```python
from build123d import *

# Parameters (mm, degrees)
F0_W     = 30
F0_H     = 30
F0_R     = 5
F1_DEPTH = 3
F0_R_2   = 4
F2_DEPTH = 6.5
F3_DEPTH = 13.5
F5_D     = 5


with BuildPart() as f1:
    # F0 (on Top) → F1 (new body)
    with BuildSketch(Plane.XY):
        Rectangle(F0_W, F0_H)
        Circle(F0_R, mode=Mode.SUBTRACT)
    extrude(amount=F1_DEPTH)

    # F0 (on Top) → F2 (join)
    with BuildSketch(Plane.XY):
        Circle(F0_R)
        Circle(F0_R_2, mode=Mode.SUBTRACT)
    extrude(amount=F2_DEPTH)

    # F0 (on Top) → F3 (join)
    with BuildSketch(Plane.XY):
        Circle(F0_R_2)
    extrude(amount=F3_DEPTH)

    # F5 (through all)
    with Locations(Plane.XY.offset(3)):
        with Locations((8.5, 8.5), (-8.5, 8.5), (-8.5, -8.5), (8.5, -8.5)):
            Hole(F5_D / 2)


with BuildPart() as f6_1:
    # F6: copy of F1
    add(f1.part.moved(Location((50, 0, 0))))


solid = f1.part
```
Read the model definition and answer for the solid it produces. Units are mm, in the model's axes. A direction names the side the tool comes from. Coordinates: 2 decimals unless noted, no trailing zeros. Loops run counter-clockwise (first coordinate to the right, second up) from the corner with the lowest first, then second, coordinate; pieces in that order, holes last. Notation, with made-up numbers: (52.5, -4.5) -> (59.5, -4.5) arc R22 cw to (59.5, 21.5) -> close; hole circle Ø10 at (-16, 30). An arc over 180 degrees is marked (long way). Return JSON: item names as keys, results as strings.
Item 1: Find section C-C (z = 1.25). Determine the outline of the cut face in (x, y).
Answers:
{"outline": "(-15, -15) -> (15, -15) -> (15, 15) -> (-15, 15) -> close; hole circle Ø5 at (-8.5, -8.5); hole circle Ø5 at (-8.5, 8.5); hole circle Ø5 at (8.5, -8.5); hole circle Ø5 at (8.5, 8.5)"}
Item 2: For faces 4 (the flat face through (0, 15, 1)), 5 (the cylindrical face through (-0.867, -3.905, 9.951)), determine the directions among +Z, -Z, +X, -X, +Y, -Y from which every point of the face is accessible in a straight line to the end or side of a thin tool.
Answers:
{"face 4": "+Z, -Z, +X, -X, +Y", "face 5": "+Z"}
Item 3: Find section D-D (x = 0). Determine the outline of the cut face in (y, z), plus the area to 3 significant figures.
Answers:
{"outline": "(-15, 0) -> (15, 0) -> (15, 3) -> (5, 3) -> (5, 6.5) -> (4, 6.5) -> (4, 13.5) -> (-4, 13.5) -> (-4, 6.5) -> (-5, 6.5) -> (-5, 3) -> (-15, 3) -> close", "area": "181 mm2"}
Item 4: Find section A-A (x = -8.5). Determine the outline of the cut face in (y, z), plus the area to 3 significant figures.
Answers:
{"outline": "(-15, 0) -> (-11, 0) -> (-11, 3) -> (-15, 3) -> close; (-6, 0) -> (6, 0) -> (6, 3) -> (-6, 3) -> close; (11, 0) -> (15, 0) -> (15, 3) -> (11, 3) -> close", "area": "60.0 mm2"}
Item 5: For a pull along Y with two mould halves and no side action, classify faces 1 (the flat face through (-4, 4, 3)), 2 (the cylindrical face through (-1.08, -4.88, 4.73)), 3 (the cylindrical face through (9.04, 6.06, 1.48)) as +Y half, -Y half, draft (parallel to the pull), parting line (faces both ways), or undercut.
Answers:
{"face 1": "draft", "face 2": "parting line", "face 3": "undercut"}
Item 6: Flat-ended cylindrical pins translate along their axes: P1, Ø5, axis at x = 12, z = 6, coming from the -Y side; P2, Ø2, axis at x = 0, z = 12, coming from the -Y side; P3, Ø5, axis at x = 11.5, y = 0, coming from the +Z side. Find the tip coordinate at first contact, or state that the pin passes through.
Answers:
{"P1": "passes through", "P2": "stops at y = -4", "P3": "stops at z = 3"}
Item 7: Find the intervals of material crossed by probe 1 along Y at (x, z) = (-8.5, 0.85); probe 2 along Z at (x, y) = (-12.5, 11.5); probe 3 along Y at (x, z) = (0.25, 8.75), in increasing order.
Answers:
{"probe 1": "y = -15 to -11, -6 to 6, 11 to 15", "probe 2": "z = 0 to 3", "probe 3": "y = -3.99 to 3.99"}
